Read the model definition and answer for the solid it produces. Units are mm, in the model's axes. A direction names the side the tool comes from. Coordinates: 2 decimals unless noted, no trailing zeros. Write each loop counter-clockwise with the first axis right and the second up, starting at its lowest first coordinate (ties: lowest second). Pieces come first, ordered by that corner, then holes. Notation, with made-up numbers: (-23, 15) -> (-13, 15) arc R25 cw to (-13, 46) -> close; hole circle Ø1 at (84, -20.75). An arc over 180 degrees is marked (long way). Use CSV: the item, a comma, the result in double quotes.
from build123d import *

# Parameters (mm, degrees)
SKETCH2_W                    = 139.7
SKETCH2_H                    = 190.5
BASE_PLATE_DEPTH             = 2.54
SKETCH5_W                    = 38.1
SKETCH5_H                    = 95.25
STEERING_WHEELS_HOLES_DEPTH  = 6.35
FILLET1_R                    = 12.7
FILLET2_R                    = 2.54
SKETCH18_R                   = 1.651
HOLES_FOR_ARDUINO_UNO_DEPTH  = 119.144134852
SKETCH20_R                   = 9.525
CUTOUT_FOR_MOTOR_WIRES_DEPTH = 119.144134852
SKETCH24_R                   = 1.57
CUT_EXTRUDE1_DEPTH           = 2.54
SKETCH25_R                   = 1.57
CUT_EXTRUDE3_DEPTH           = 2.54
SKETCH27_W                   = 91.44
SKETCH27_H                   = 3.14
CUT_EXTRUDE4_DEPTH           = 2.54
SKETCH28_W                   = 38.1
SKETCH28_H                   = 25.4
BOSS_EXTRUDE1_DEPTH          = 2.54
SKETCH29_R                   = 6
CUT_EXTRUDE5_DEPTH           = 119.144134852
SKETCH30_W                   = 17.78
SKETCH30_H                   = 40.132
CUT_EXTRUDE6_DEPTH           = 119.144134852
CUT_EXTRUDE7_DEPTH           = 2.54


with BuildPart() as part:
    # Sketch2 → Base Plate (new body)
    with BuildSketch(Plane(origin=(0, 0, 0), x_dir=(1, 0, 0), z_dir=(0, 1, 0))):
        Rectangle(SKETCH2_W, SKETCH2_H)
    extrude(amount=BASE_PLATE_DEPTH)

    # Sketch5 → Steering Wheels Holes (cut)
    with BuildSketch(Plane(origin=(0, 2.54, 0), x_dir=(1, 0, 0), z_dir=(0, 1, 0))):
        with Locations((-50.8, 22.225)):
            Rectangle(SKETCH5_W, SKETCH5_H)
        with Locations((50.8, 22.225)):
            Rectangle(SKETCH5_W, SKETCH5_H)
    extrude(amount=-STEERING_WHEELS_HOLES_DEPTH, mode=Mode.SUBTRACT)

    # Fillet1
    fillet1_edges = [part.edges().sort_by_distance(p)[0] for p in [
        (69.85, 1.27, 95.25),
        (-69.85, 1.27, 95.25),
        (-69.85, 1.27, -95.25),
        (69.85, 1.27, -95.25),
    ]]
    fillet(fillet1_edges, radius=FILLET1_R)

    # Fillet2
    fillet2_edges = [part.edges().sort_by_distance(p)[0] for p in [
        (-69.85, 1.27, 25.4),
        (-69.85, 1.27, -69.85),
        (69.85, 1.27, -69.85),
        (69.85, 1.27, 25.4),
    ]]
    fillet(fillet2_edges, radius=FILLET2_R)

    # Sketch18 → Holes for Arduino UNO (cut, through all)
    with BuildSketch(Plane(origin=(0, 2.54, 0), x_dir=(1, 0, 0), z_dir=(0, 1, 0))):
        with Locations(Location((-8.763, -19.05, 0), (0, 0, 270))):
            Circle(SKETCH18_R)
        with Locations(Location((19.177, -19.05, 0), (0, 0, 270))):
            Circle(SKETCH18_R)
        with Locations(Location((-24.003, -69.85, 0), (0, 0, 270))):
            Circle(SKETCH18_R)
        with Locations(Location((24.309664393, -71.12, 0), (0, 0, 270))):
            Circle(SKETCH18_R)
    extrude(amount=-HOLES_FOR_ARDUINO_UNO_DEPTH, mode=Mode.SUBTRACT)

    # Sketch20 → Cutout for motor wires (cut, through all)
    with BuildSketch(Plane(origin=(0, 2.54, 0), x_dir=(1, 0, 0), z_dir=(0, 1, 0))):
        with Locations(Location((0, -5.08, 0), (0, 0, 270))):
            Circle(SKETCH20_R)
    extrude(amount=-CUTOUT_FOR_MOTOR_WIRES_DEPTH, mode=Mode.SUBTRACT)

    # Sketch24 → Cut-Extrude1 (cut)
    with BuildSketch(Plane(origin=(0, 2.54, 0), x_dir=(1, 0, 0), z_dir=(0, 1, 0))):
        with Locations(Location((-59.69, 85.09, 0), (0, 0, 270))):
            Circle(SKETCH24_R)
    cut_extrude1 = extrude(amount=-CUT_EXTRUDE1_DEPTH, mode=Mode.SUBTRACT)

    # Mirror1: Cut-Extrude1 across plane
    add(cut_extrude1.mirror(Plane(origin=(0, 0, 0), x_dir=(0, 0, 1), z_dir=(1, 0, 0))), mode=Mode.SUBTRACT)

    # Sketch25 → Cut-Extrude3 (cut)
    with BuildSketch(Plane(origin=(0, 2.54, 0), x_dir=(1, 0, 0), z_dir=(0, 1, 0))):
        with Locations(Location((-59.69, -85.09, 0), (0, 0, 270))):
            Circle(SKETCH25_R)
        with Locations(Location((59.69, -85.09, 0), (0, 0, 90))):
            Circle(SKETCH25_R)
    extrude(amount=-CUT_EXTRUDE3_DEPTH, mode=Mode.SUBTRACT)

    # Sketch27 → Cut-Extrude4 (cut)
    with BuildSketch(Plane(origin=(0, 2.54, 0), x_dir=(1, 0, 0), z_dir=(0, 1, 0))):
        with Locations((0, -85.09)):
            Rectangle(SKETCH27_W, SKETCH27_H)
        with Locations((0, 85.09)):
            Rectangle(SKETCH27_W, SKETCH27_H)
    extrude(amount=-CUT_EXTRUDE4_DEPTH, mode=Mode.SUBTRACT)

    # Sketch28 → Boss-Extrude1 (add, through all)
    with BuildSketch(Plane(origin=(0, 2.54, 0), x_dir=(1, 0, 0), z_dir=(0, 1, 0))):
        with Locations((-50.8, 22.225)):
            Rectangle(SKETCH28_W, SKETCH28_H)
    boss_extrude1 = extrude(amount=-BOSS_EXTRUDE1_DEPTH)

    # Mirror2: Boss-Extrude1 across plane
    add(boss_extrude1.mirror(Plane(origin=(0, 0, 0), x_dir=(0, 0, 1), z_dir=(1, 0, 0))))

    # Sketch29 → Cut-Extrude5 (cut, through all)
    with BuildSketch(Plane.XZ):
        with Locations(Location((-57.3106296, -21.945186919, 0), (0, 0, 270))):
            Circle(SKETCH29_R)
    cut_extrude5 = extrude(amount=-CUT_EXTRUDE5_DEPTH, mode=Mode.SUBTRACT)

    # Mirror3: Cut-Extrude5 across plane
    add(cut_extrude5.mirror(Plane(origin=(0, 0, 0), x_dir=(0, 0, 1), z_dir=(1, 0, 0))), mode=Mode.SUBTRACT)

    # Sketch30 → Cut-Extrude6 (cut, through all)
    with BuildSketch(Plane.XZ):
        with Locations((0, -33.375186919)):
            Rectangle(SKETCH30_W, SKETCH30_H)
    extrude(amount=-CUT_EXTRUDE6_DEPTH, mode=Mode.SUBTRACT)

    # Sketch31 → Cut-Extrude7 (cut)
    with BuildSketch(Plane.XZ):
        Polygon((-66.782826822, 33.314746009), (-27.963596323, 33.314746009), (-27.963596323, 37.60631923), (-44.154531657, 37.60631923), (-27.963596323, 43.848607552), (-29.63125682, 48.174101966), (-47.373211572, 41.333830254), (-65.115166325, 48.174101966), (-66.782826822, 43.848607552), (-50.591891488, 37.60631923), (-66.782826822, 37.60631923), align=None)
        Polygon((31.121508027, 33.314746009), (36.190157542, 33.314746009), (36.190157542, 48.174101966), (62.547135024, 48.174101966), (62.547135024, 54.772612114), (36.190157542, 54.772612114), (36.190157542, 69.200784581), (31.121508027, 69.200784581), align=None)
    extrude(amount=-CUT_EXTRUDE7_DEPTH, mode=Mode.SUBTRACT)


solid = part.part
1. A tool of negligible diameter and unlimited length cuts with its end or side. For faces 4 (the flat face through (-56.1, 1.3, 44.7)), 5 (the cylindrical face through (66.03, 1.29, 91.63)), from which of +Z, -Z, +X, -X, +Y, -Y can it reach the whole face along a straight path? Write none if from no direction.
Solutions:
face 4,"+Y, -Y"
face 5,"+Z, +X, +Y, -Y"
2. Find the intervals of material crossed by line 1 along X through (y, z) = (0.6, 19.05); line 2 along Z through (x, y) = (22.5, 1.95); line 3 along Z through (x, y) = (40.5, 1.45) (3 decimals), in increasing order.
Solutions:
line 1,"x = -31.75 to -10.41, -7.11 to 17.53, 20.83 to 31.75"
line 2,"z = -95.25 to -86.66, -83.52 to 83.52, 86.66 to 95.25"
line 3,"z = -95.25 to -86.66, -83.52 to -69.85, -34.925 to -9.525, 25.4 to 48.174, 54.773 to 83.52, 86.66 to 95.25"
3. A cutting plane is placed at A-A (z = 5.08). Give the vertices of the cut face in (x, y) (3 decimals), and give its area (3 significant figures).
Solutions:
outline,"(-31.75, 0) -> (-9.525, 0) -> (-9.525, 2.54) -> (-31.75, 2.54) -> close; (9.525, 0) -> (31.75, 0) -> (31.75, 2.54) -> (9.525, 2.54) -> close"
area,"113 mm^2"
4. A cutting plane is placed at B-B (x = 0). Give the vertices of the cut face in (y, z) (3 decimals).
Solutions:
outline,"(0, -95.25) -> (2.54, -95.25) -> (2.54, -86.66) -> (0, -86.66) -> close; (0, -83.52) -> (2.54, -83.52) -> (2.54, -53.441) -> (0, -53.441) -> close; (0, -13.309) -> (2.54, -13.309) -> (2.54, -4.445) -> (0, -4.445) -> close; (0, 14.605) -> (2.54, 14.605) -> (2.54, 83.52) -> (0, 83.52) -> close; (0, 86.66) -> (2.54, 86.66) -> (2.54, 95.25) -> (0, 95.25) -> close"
5. A cutting plane is placed at C-C (z = 52). Give the vertices of the cut face in (x, y), and give its area (3 significant figures).
Solutions:
outline,"(-69.85, 0) -> (31.12, 0) -> (31.12, 2.54) -> (-69.85, 2.54) -> close; (62.55, 0) -> (69.85, 0) -> (69.85, 2.54) -> (62.55, 2.54) -> close"
area,"275 mm^2"
6. A cutting plane is placed at D-D (y = 0.8). Give the number of separate pieces and of enclosed holes in the cut face, and give its area (3 significant figures).
Solutions:
separate pieces,"1"
enclosed holes,"16"
area,"18,600 mm^2"
7. For a pull along X with two mould halves and no side action, classify faces 1 (the cylindrical face through (-66.23, 1.29, 91.43)), 2 (the cylindrical face through (66.03, 1.29, -91.63)), 3 (the cylindrical face through (-63.168, 1.252, -20.645)) as pulls with the +X half, pulls with the -X half, needs draft (parallel to the pull), parting line crosses it, or undercut.
Solutions:
face 1,"pulls with the -X half"
face 2,"pulls with the +X half"
face 3,"undercut"
